Design review of the part shown in the three views and the two pictorial views. Dimensions are in mm from the part's minimum x, y and z. Round coordinates to 2 decimals unless told otherwise and drop trailing zeros. Write each loop counter-clockwise with the first axis right and the second up, starting at its lowest first coordinate (ties: lowest second). Pieces come first, ordered by that corner, then holes. Notation, with made-up numbers: (28.25, 50.25) -> (82.25, 50.25) arc R20 ccw to (82.25, 83.25) -> close; hole circle Ø3 at (63.5, 65.25). An arc over 180 degrees is marked (long way). Answer as a JSON object with one key per item and string values. Group by question number.
1) Insertion check: pin 1 Ø1.5 at (x, z) = (27, 17) entering from -Y; pin 2 Ø3 at (x, y) = (79.5, 13.5) entering from +Z; pin 3 Ø6 at (x, z) = (44, 34.5) entering from +Y; pin 4 Ø1 at (y, z) = (46, 52) entering from -X. Each pin has a flat end and moves straight along its axis. Give the tip position at first contact, or say it passes through.
2) To check wall thickness, follow probe 1 along Y at (x, z) = (64, 39); probe 2 along X at (y, z) = (15, 67.5) (1 decimal); probe 3 along Y at (x, z) = (23.5, 13). State the ranges of each line that lie inside material, in increasing order. Write a range as [from, to].
3) Mouldability with a two-part tool opening along Y and no side actions: class the marked faces 1, 2 and 3 as pulls with the +Y half, pulls with the -Y half, needs draft (parallel to the pull), parting line crosses it, or undercut.
4) We need section C-C, the plane z = 53.5. Write out the cut boundary in (x, y), then the cut area to 3 significant figures.
5) We need section A-A, the plane x = 76.5. Write out the cut boundary in (y, z).
6) We need section B-B, the plane y = 79. Write out the cut boundary in (x, z), then the cut area to 3 significant figures.
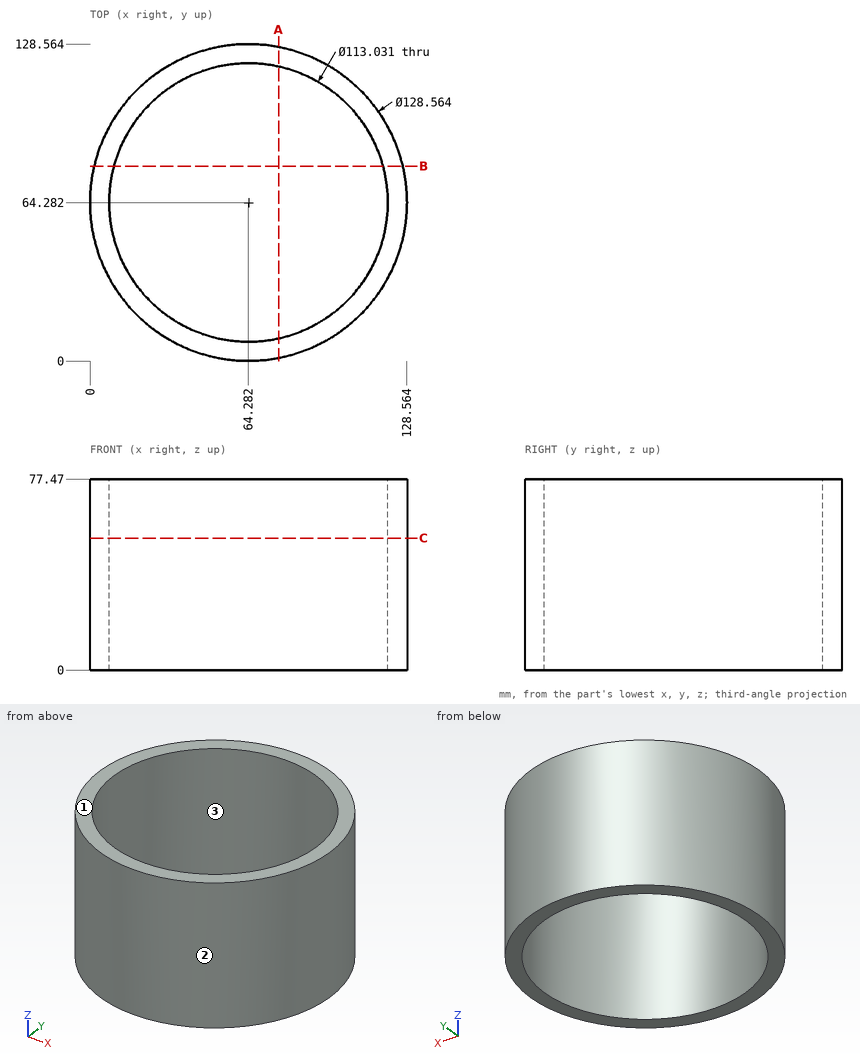
Here are the results:
{
 "1": {"pin 1": "stops at y = 11.39", "pin 2": "passes through", "pin 3": "stops at y = 126.2", "pin 4": "stops at x = 2.51"},
 "2": {"probe 1": "y = [0, 7.77], [120.8, 128.56]", "probe 2": "x = [23, 36.6], [91.9, 105.6]", "probe 3": "y = [14.59, 25.16], [103.41, 113.97]"},
 "3": {"face 1": "needs draft", "face 2": "parting line crosses it", "face 3": "undercut"},
 "4": {"outline": "circle Ø128.56 at (64.28, 64.28); hole circle Ø113.03 at (64.28, 64.28)", "area": "2,950 mm^2"},
 "5": {"outline": "(1.17, 0) -> (9.1, 0) -> (9.1, 77.47) -> (1.17, 77.47) -> close; (119.46, 0) -> (127.39, 0) -> (127.39, 77.47) -> (119.46, 77.47) -> close"},
 "6": {"outline": "(1.71, 0) -> (9.72, 0) -> (9.72, 77.47) -> (1.71, 77.47) -> close; (118.85, 0) -> (126.86, 0) -> (126.86, 77.47) -> (118.85, 77.47) -> close", "area": "1,240 mm^2"}
}
